Build history of the part. All positions in model axes, mm. Face numbers are marked on the shaded views. A direction names the side the tool comes from. Give positions to 0.01 mm unless a question says otherwise; leave off trailing zeros. Loops run counter-clockwise (first coordinate to the right, second up) from the corner with the lowest first, then second, coordinate; pieces in that order, holes last. Notation, with made-up numbers: (13, 57.25) -> (30, 57.25) arc R29 cw to (30, 83.25) -> close; hole circle Ø8 at (-19, -26.75). An arc over 180 degrees is marked (long way). Answer in a Markdown table with one row per item. Add a question column.
from build123d import *

# Parameters (mm, degrees)
F0_W = 12.7
F0_H = 11.90625


with BuildPart() as f1:
    # F0 (on Front) → F1 (revolve)
    with BuildSketch(Plane.XZ):
        with BuildLine():
            Line((-12.7, 11.90625), (-12.7, 0))
            Line((-12.7, 0), (12.7, 0))
            Line((12.7, 0), (12.7, 11.90625))
            Line((12.7, 11.90625), (12.7, 25.4))
            Line((12.7, 25.4), (11.219473, 22.225))
            ThreePointArc((11.219473, 22.225), (6.650816, 17.023914), (0, 15.102826))
            ThreePointArc((0, 15.102826), (-6.650816, 17.023914), (-11.219473, 22.225))
            Line((-11.219473, 22.225), (-12.7, 25.4))
            Line((-12.7, 25.4), (-12.7, 11.90625))
        make_face()
        with Locations((-19.05, 5.953125)):
            Rectangle(F0_W, F0_H)
        with Locations((19.05, 5.953125)):
            Rectangle(F0_W, F0_H)
    revolve(axis=Axis((0, 0, 0), (1, 0, 0)))


solid = f1.part
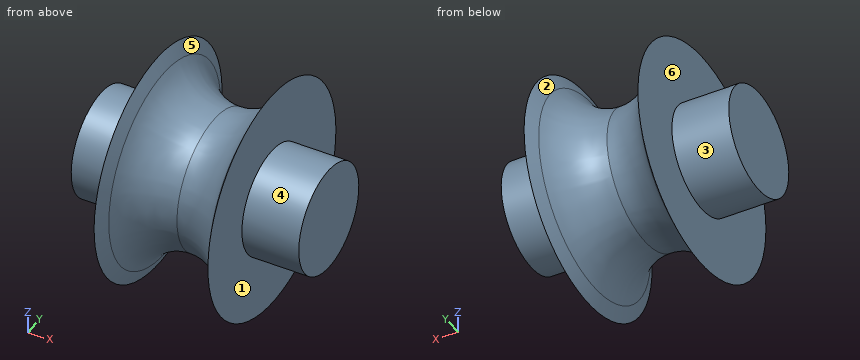
(1) 3-axis set-ups, long thin cutter, end or side, ignore diameter. For the marked faces 1, 2 and 3: which of +Z, -Z, +X, -X, +Y, -Y reach the whole face in a straight line?
(2) Saw through at D-D, the plane x = 4.5. List the corners of the cut face in (y, z), then the cut area to 3 significant figures.
(3) Two-plate mould, pull along X, no slides. Class the marked faces 4, 5 and 6: released by +X, released by -X, zero draft, split by the parting line, or undercut.
(4) Saw through at A-A, the plane z = 0. List the corners of the cut face in (x, y) (3 decimals).
(5) Wall check: line 1 along X through (y, z) = (2.5, 13.5); line 2 along X through (y, z) = (18.5, 4); line 3 along X through (y, z) = (1, 23). Give the ranges that are in metal, low to high. Write a range as from..to.
(6) Flat gauge pins, fed straight in: pin 1 Ø8 at (y, z) = (7.5, 19) entering from -X; pin 2 Ø12 at (x, z) = (-7.5, 1.5) entering from +Y; pin 3 Ø5 at (x, z) = (-2, 4.5) entering from +Y. Where does each tip first touch, or does it go through?
(7) Saw through at C-C, the plane x = -7.5. List the corners of the cut face in (y, z).
Worked answers:
| question | item | result |
|---|---|---|
| 1 | face 1 | +X |
| 1 | face 2 | none |
| 1 | face 3 | -X |
| 2 | outline | circle Ø31.87 at (0, 0) |
| 2 | area | 798 mm^2 |
| 3 | face 4 | zero draft |
| 3 | face 5 | undercut |
| 3 | face 6 | released by -X |
| 4 | outline | (-25.4, -11.906) -> (-12.7, -11.906) -> (-12.7, -25.4) -> (-11.219, -22.225) arc R12.335 cw to (0, -15.103) arc R12.335 cw to (11.219, -22.225) -> (12.7, -25.4) -> (12.7, -11.906) -> (25.4, -11.906) -> (25.4, 11.906) -> (12.7, 11.906) -> (12.7, 25.4) -> (11.219, 22.225) arc R12.335 cw to (0, 15.103) arc R12.335 cw to (-11.219, 22.225) -> (-12.7, 25.4) -> (-12.7, 11.906) -> (-25.4, 11.906) -> close |
| 5 | line 1 | -12.7..12.7 |
| 5 | line 2 | -12.7..-8.97, 8.97..12.7 |
| 5 | line 3 | -12.7..-11.59, 11.59..12.7 |
| 6 | pin 1 | x = -12.7 |
| 6 | pin 2 | y = 25.4 |
| 6 | pin 3 | y = 15.48 |
| 7 | outline | circle Ø35.23 at (0, 0) |
